```python
from build123d import *

# Parameters (mm, degrees)
F0_W     = 142
F0_H     = 34
F1_DEPTH = 10
F3_D     = 4.4
F4_SIZE  = 10
F5_R     = 5


with BuildPart() as f1:
    # F0 (on Top) → F1 (new body)
    with BuildSketch(Plane.XY):
        Rectangle(F0_W, F0_H)
    extrude(amount=F1_DEPTH)

    # F3 (through all)
    with Locations(Plane.XY.offset(10)):
        with Locations((-56, 0), (-24, 0), (24, 0), (56, 0)):
            Hole(F3_D / 2)

    # F4
    f4_edges = [f1.edges().sort_by_distance(p)[0] for p in [
        (-71, -17, 5),
        (71, -17, 5),
        (71, 17, 5),
        (-71, 17, 5),
    ]]
    chamfer(f4_edges, length=F4_SIZE)

    # F5
    f5_edges = [f1.edges().sort_by_distance(p)[0] for p in [
        (-61, -17, 5),
        (-71, -7, 5),
        (61, -17, 5),
        (71, -7, 5),
        (71, 7, 5),
        (61, 17, 5),
        (-61, 17, 5),
        (-71, 7, 5),
    ]]
    fillet(f5_edges, radius=F5_R)


solid = f1.part
```
Part model, mm, in its own coordinate system. Round coordinates to 2 decimals unless told otherwise and drop trailing zeros. Write each loop counter-clockwise with the first axis right and the second up, starting at its lowest first coordinate (ties: lowest second). Pieces come first, ordered by that corner, then holes. Notation, with made-up numbers: M 85.25,-33.75 L 133.25,-33.75 A28 ccw 133.25,-10.75 Z; hole C 49.5,64 d4. An arc over 180 degrees is marked long. Answer as CSV lines item,"result". Start each with the question number.
1) Band-saw the part on B-B (z = 8.75). List the corners of the cut face in (x, y), then the cut area to 3 significant figures.
2) Drill centre lines: L1, parallel to Y at x = -56, z = 6; L2, parallel to X at y = 5, z = 3.25; L3, parallel to X at y = 1, z = 1.5. Where is each one in solid material? Low to high.
3) Mould opens along X. For faces 1 (the face through (-26.032, -0.843, 4.93)), 2 (the face through (60.82, -16.63, 5.07)), 3 (the face through (-53.802, 0.097, 4.93)), 4 (the face through (-1, 0, 0)) say: +X half, -X half, draft (parallel to the pull), parting line (faces both ways), or undercut.
4) Band-saw the part on D-D (y = -10.5). List the corners of the cut face in (x, z), then the cut area to 3 significant figures.
5) Drop a flat-ended pin along its axis: pin 1 (6 mm diameter, centred on y = 12, z = 8.5, fed in from +X). Give the stop position or say it passes through.
6) Band-saw the part on A-A (x = 24). List the corners of the cut face in (y, z).
7) Band-saw the part on C-C (y = 0). List the corners of the cut face in (x, z).
Worked out:
1,outline,"M -71,-4.93 A5 ccw -69.54,-8.46 L -62.46,-15.54 A5 ccw -58.93,-17 L 58.93,-17 A5 ccw 62.46,-15.54 L 69.54,-8.46 A5 ccw 71,-4.93 L 71,4.93 A5 ccw 69.54,8.46 L 62.46,15.54 A5 ccw 58.93,17 L -58.93,17 A5 ccw -62.46,15.54 L -69.54,8.46 A5 ccw -71,4.93 Z; hole C -56,0 d4.4; hole C -24,0 d4.4; hole C 24,0 d4.4; hole C 56,0 d4.4"
1,area,"4,560 mm²"
2,L1,"-17 to -2.2, 2.2 to 17"
2,L2,"-71 to 71"
2,L3,"-71 to -57.96, -54.04 to -25.96, -22.04 to 22.04, 25.96 to 54.04, 57.96 to 71"
3,face 1,"undercut"
3,face 2,"+X half"
3,face 3,"undercut"
3,face 4,"draft"
4,outline,"M -67.5,0 L 67.5,0 L 67.5,10 L -67.5,10 Z"
4,area,"1,350 mm²"
5,pin 1,"x = 69"
6,outline,"M -17,0 L -2.2,0 L -2.2,10 L -17,10 Z; M 2.2,0 L 17,0 L 17,10 L 2.2,10 Z"
7,outline,"M -71,0 L -58.2,0 L -58.2,10 L -71,10 Z; M -53.8,0 L -26.2,0 L -26.2,10 L -53.8,10 Z; M -21.8,0 L 21.8,0 L 21.8,10 L -21.8,10 Z; M 26.2,0 L 53.8,0 L 53.8,10 L 26.2,10 Z; M 58.2,0 L 71,0 L 71,10 L 58.2,10 Z"
